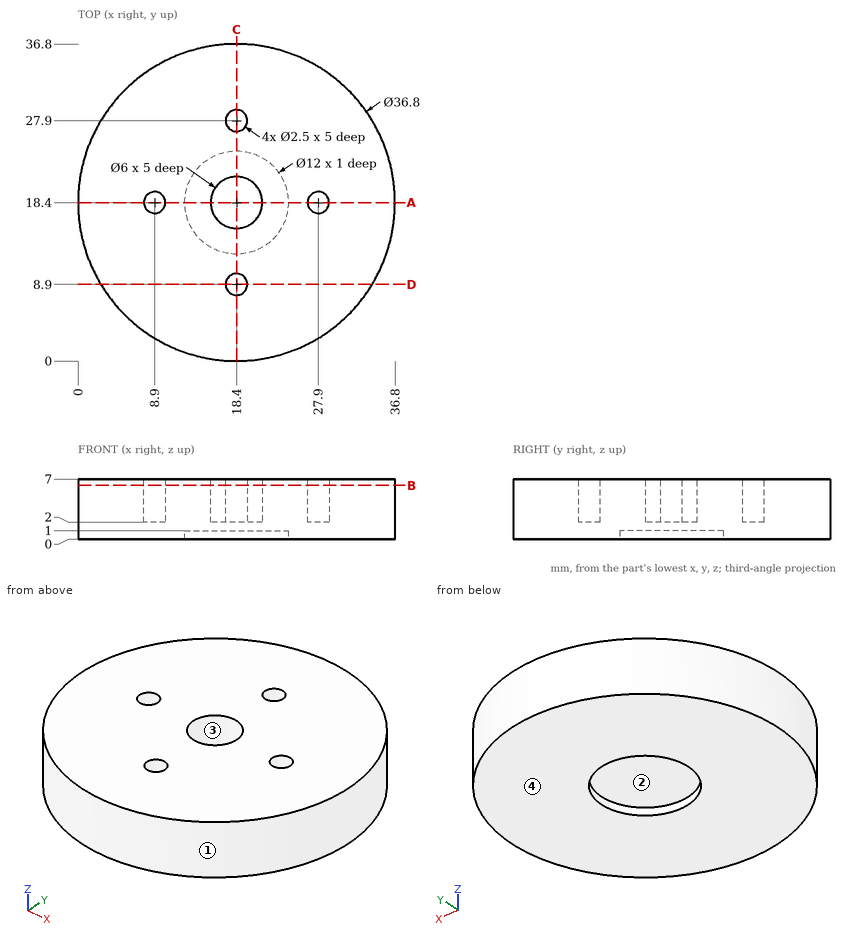
Study the drawing (mm; zero at the part's minimum x, y, z) and answer. Round coordinates to 2 decimals unless told otherwise and drop trailing zeros. Loops run counter-clockwise (first coordinate to the right, second up) from the corner with the lowest first, then second, coordinate; pieces in that order, holes last. Notation, with made-up numbers: (16, 67) -> (60, 67) arc R27 cw to (60, 103) -> close; hole circle Ø6 at (65, -11.75). An arc over 180 degrees is marked (long way). One line per item, written item: value.
1) Consider L1, parallel to Y at x = 18.4, z = 5.5; L2, parallel to Y at x = 18.4, z = 0.2; L3, parallel to Y at x = 17.5, z = 5.25. Determine where each line is inside the solid, lowest interval first. Write a range as [from, to].
Answer list:
L1: y = [0, 7.65], [10.15, 15.4], [21.4, 26.65], [29.15, 36.8]
L2: y = [0, 12.4], [24.4, 36.8]
L3: y = [0.02, 8.03], [9.77, 15.54], [21.26, 27.03], [28.77, 36.78]
2) Flat-ended cylindrical pins translate along their axes: P1, Ø3, axis at y = 24, z = 2, coming from the +X side; P2, Ø3, axis at x = 19.5, y = 18.5, coming from the +Z side; P3, Ø4, axis at x = 7, z = 4.5, coming from the -Y side. Find the tip coordinate at first contact, or state that the pin passes through.
Answer list:
P1: stops at x = 36.34
P2: stops at z = 2
P3: stops at y = 2.58
3) A cutting plane is placed at B-B (z = 6.25). Determine the outline of the cut face in (x, y).
Answer list:
outline: circle Ø36.8 at (18.4, 18.4); hole circle Ø2.5 at (8.9, 18.4); hole circle Ø6 at (18.4, 18.4); hole circle Ø2.5 at (18.4, 8.9); hole circle Ø2.5 at (18.4, 27.9); hole circle Ø2.5 at (27.9, 18.4)
4) The mould has two halves that part along Y. Classify the marked faces 1, 2, 3 and 4: pulls with the +Y half, pulls with the -Y half, needs draft (parallel to the pull), parting line crosses it, or undercut.
Answer list:
face 1: parting line crosses it
face 2: undercut
face 3: undercut
face 4: needs draft
5) A cutting plane is placed at A-A (y = 18.4). Determine the outline of the cut face in (x, z), and give its area (3 significant figures).
Answer list:
outline: (0, 0) -> (12.4, 0) -> (12.4, 1) -> (24.4, 1) -> (24.4, 0) -> (36.8, 0) -> (36.8, 7) -> (29.15, 7) -> (29.15, 2) -> (26.65, 2) -> (26.65, 7) -> (21.4, 7) -> (21.4, 2) -> (15.4, 2) -> (15.4, 7) -> (10.15, 7) -> (10.15, 2) -> (7.65, 2) -> (7.65, 7) -> (0, 7) -> close
area: 191 mm²
6) A cutting plane is placed at D-D (y = 8.9). Determine the outline of the cut face in (x, z).
Answer list:
outline: (2.64, 0) -> (34.16, 0) -> (34.16, 7) -> (19.65, 7) -> (19.65, 2) -> (17.15, 2) -> (17.15, 7) -> (2.64, 7) -> close
